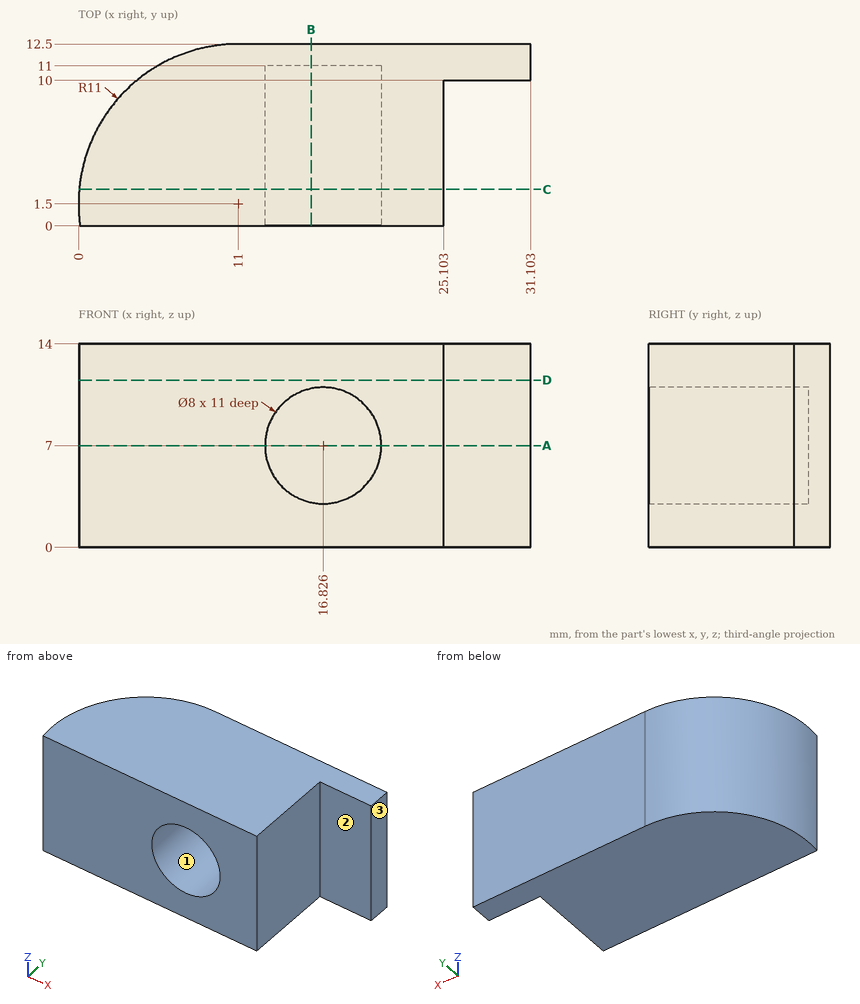
Can you work these out from the drawing? Everything is in mm from the part's minimum corner. A direction names the side the tool comes from. Round coordinates to 2 decimals unless told otherwise and drop trailing zeros. Order: outer loops, then holes, each group sorted by start corner. A loop starts at its lowest first (then second) coordinate and runs counter-clockwise, first axis right, second up.
(1) If I drill on L1, parallel to X at y = 1.5, z = 7 (1 decimal); L2, parallel to X at y = 5.5, z = 7 (1 decimal); L3, parallel to Y at x = 25.5, z = 4.5, over which ranges is the centre line in solid material (lowest first)?
Results are:
L1: x = 0 to 12.8, 20.8 to 25.1
L2: x = 0.8 to 12.8, 20.8 to 25.1
L3: y = 10 to 12.5
(2) On a 3-axis mill with a long thin cutter (end or side, diameter ignored), from which of +Z, -Z, +X, -X, +Y, -Y can I reach the whole of each face in a straight line? I mean the marked faces 1, 2 and 3. Say none if no direction works.
Results are:
face 1: -Y
face 2: +Z, -Z, +X, -Y
face 3: +Z, -Z, +X, +Y, -Y
(3) If we section it at D-D (z = 11.5): Please give me the cut outline in (x, y), plus the area to 3 significant figures.
Results are:
outline: (0.1, 0) - (25.1, 0) - (25.1, 10) - (31.1, 10) - (31.1, 12.5) - (11, 12.5) arc R11 ccw to start
area: 303 mm2
(4) If we section it at A-A (z = 7): Please give me the cut outline in (x, y) (1 decimal).
Results are:
outline: (0.1, 0) - (12.8, 0) - (12.8, 11) - (20.8, 11) - (20.8, 0) - (25.1, 0) - (25.1, 10) - (31.1, 10) - (31.1, 12.5) - (11, 12.5) arc R11 ccw to start
(5) I'm going to push flat-ended pins straight in: pin 1 (6 mm diameter, centred on y = 4, z = 5.5, fed in from -X); pin 2 (5 mm diameter, centred on y = 2.5, z = 6, fed in from +X); pin 3 (3 mm diameter, centred on x = 29, z = 6.5, fed in from -Y); pin 4 (2 mm diameter, centred on y = 8, z = 1.5, fed in from -X) (1 decimal). Where does each tip first touch, or does it pass through?
Results are:
pin 1: stops at x = 0
pin 2: stops at x = 25.1
pin 3: stops at y = 10
pin 4: stops at x = 1.5
(6) If we section it at C-C (y = 2.5): Please give me the cut outline in (x, z) (1 decimal).
Results are:
outline: (0, 0) - (25.1, 0) - (25.1, 14) - (0, 14) - close; hole circle Ø8 at (16.8, 7)
(7) If we section it at B-B (x = 16): Please give me the cut outline in (y, z).
Results are:
outline: (0, 0) - (12.5, 0) - (12.5, 14) - (0, 14) - (0, 10.91) - (11, 10.91) - (11, 3.09) - (0, 3.09) - close
